Geometry check sheet. Reference: the model listing, model coordinates, mm. Coordinates: 2 decimals unless noted, no trailing zeros. Write each loop counter-clockwise with the first axis right and the second up, starting at its lowest first coordinate (ties: lowest second). Pieces come first, ordered by that corner, then holes. Notation, with made-up numbers: (20, 40.25) -> (62, 40.25) arc R9 cw to (62, 57.25) -> close; hole circle Ø10 at (36, 29). An arc over 180 degrees is marked (long way). Use a Markdown table: item, result.
Autodesk Inventor part; units mm, degrees
ref_plane "YZ Plane" through (0, 0, 0) normal (1, 0, 0) x (0, 1, 0)
ref_plane "XZ Plane" through (0, 0, 0) normal (0, 1, 0) x (-1, 0, 0)
ref_plane "XY Plane" through (0, 0, 0) normal (0, 0, 1) x (1, 0, 0)
sketch "Sketch1" plane through (0, 0, 0) normal (0, 0, 1) x (1, 0, 0)
  line L0 (0, 37.2) -> (5, 42.2)
  line L1 (37.2, 42.2) -> (42.2, 37.2)
  line L2 (42.2, 5) -> (37.2, 0)
  line L3 (5, 0) -> (0, 5)
  line L4 (0, 37.2) -> (0, 5)
  line L5 (37.2, 42.2) -> (5, 42.2)
  line L6 (42.2, 5) -> (42.2, 37.2)
  line L7 (5, 0) -> (37.2, 0)
  line L8 (0, 5) -> (0, 0)
  circle A0 centre (21.1, 21.1) radius 2.5
  circle A1 centre (5.6, 36.6) radius 1.5
  circle A2 centre (36.6, 36.6) radius 1.5
  circle A3 centre (36.6, 5.6) radius 1.5
  circle A4 centre (5.6, 5.6) radius 1.5
  dimension "d8" = 5
  dimension "d9" = 5
  dimension "d10" = 5
  dimension "d11" = 21.1
  dimension "d12" = 21.1
  dimension "d13" = 3
  dimension "d14" = 3
  dimension "d15" = 3
  dimension "d16" = 3
  dimension "d17" = 31
  dimension "d18" = 31
  dimension "d19" = 31
  dimension "d20" = 31
  dimension "d21" = 5.6
  dimension "d22" = 5.6
  dimension "d43" = 5.6
  dimension "d44" = 5.6
  dimension "d45" = 5.6
  dimension "d46" = 5.6
  dimension "d47" = 42.2
extrude "Extrusion1" add sketch "Sketch1" along normal blind 9.8
sketch "Sketch2" plane through (0, 0, 9.8) normal (0, 0, 1) x (1, 0, 0)
  circle A0 centre (21.1, 21.1) radius 2.5
  circle A1 centre (5.6, 5.6) radius 1.5
  circle A2 centre (36.6, 5.6) radius 1.5
  circle A3 centre (36.6, 36.6) radius 1.5
  circle A4 centre (5.6, 36.6) radius 1.5
  line L0 (5, 42.2) -> (0, 37.2)
  line L1 (0, 37.2) -> (0, 5)
  line L2 (0, 5) -> (5, 0)
  line L3 (5, 0) -> (37.2, 0)
  line L4 (37.2, 0) -> (42.2, 5)
  line L5 (42.2, 5) -> (42.2, 37.2)
  line L6 (42.2, 37.2) -> (37.2, 42.2)
  line L7 (37.2, 42.2) -> (5, 42.2)
  point P0 (0, 0)
fillet "Fillet1" radius 0.25 8 edges at (21.1, 42.2, 9.8) (39.7, 39.7, 9.8) (42.2, 21.1, 9.8) (39.7, 2.5, 9.8) (21.1, 0, 9.8) (2.5, 2.5, 9.8) (0, 21.1, 9.8) (2.5, 39.7, 9.8)
extrude "Extrusion2" add sketch "Sketch2" along normal blind 31
sketch "Sketch3" plane through (0, 0, 40.8) normal (0, 0, 1) x (1, 0, 0)
  circle A0 centre (21.1, 21.1) radius 2.5
  circle A1 centre (5.6, 36.6) radius 1.5
  circle A2 centre (36.6, 36.6) radius 1.5
  circle A3 centre (36.6, 5.6) radius 1.5
  circle A4 centre (5.6, 5.6) radius 1.5
  line L0 (5, 42.2) -> (0, 37.2)
  line L1 (0, 37.2) -> (0, 5)
  line L2 (0, 5) -> (5, 0)
  line L3 (5, 0) -> (37.2, 0)
  line L4 (37.2, 0) -> (42.2, 5)
  line L5 (42.2, 5) -> (42.2, 37.2)
  line L6 (42.2, 37.2) -> (37.2, 42.2)
  line L7 (37.2, 42.2) -> (5, 42.2)
  point P0 (0, 0)
fillet "Fillet2" radius 0.25 8 edges at (21.1, 42.2, 40.8) (39.7, 39.7, 40.8) (42.2, 21.1, 40.8) (39.7, 2.5, 40.8) (21.1, 0, 40.8) (2.5, 2.5, 40.8) (0, 21.1, 40.8) (2.5, 39.7, 40.8)
extrude "Extrusion3" add sketch "Sketch3" along normal blind 7.75
sketch "Sketch4" plane through (0, 0, 48.55) normal (0, 0, 1) x (1, 0, 0)
  circle A0 centre (21.1, 21.1) radius 2.5
  circle A1 centre (21.1, 21.1) radius 16
  point P0 (0, 0)
  dimension "d31" = 32
extrude "Extrusion4" cut sketch "Sketch4" against normal blind 0.6
sketch "Sketch5" plane through (21.1, 21.1, 47.95) normal (0, 0, 1) x (1, 0, 0)
  circle A0 centre (0, 0) radius 2.5
  circle A1 centre (0, 0) radius 16
  circle A2 centre (0, 0) radius 11
  point P0 (-21.1, -21.1)
  dimension "d35" = 22
extrude "Extrusion5" add sketch "Sketch5" along normal blind 2.2 contours A2
fillet "Fillet3" radius 0.5 1 edges at (10.1, 21.1, 50.15)
sketch "Sketch6" plane through (21.1, 21.1, 50.15) normal (0, 0, 1) x (1, 0, 0)
  circle A0 centre (0, 0) radius 2.5
  point P0 (-21.1, -21.1)
extrude "Extrusion6" add sketch "Sketch6" along normal blind 22.5
fillet "Fillet4" radius 0.5 1 edges at (18.6, 21.1, 72.65)
sketch "Sketch7" plane through (21.1, 21.1, 72.65) normal (0, 0, 1) x (1, 0, 0)
  circle A0 centre (0, 0) radius 2.6386
  point P0 (-21.1, -21.1)
extrude "Extrusion7" add sketch "Sketch7" along normal blind 15
sketch "Sketch8" plane through (21.1, 21.1, 87.65) normal (0, 0, 1) x (1, 0, 0)
  circle A0 centre (0, 0) radius 2
  circle A1 centre (0, 0) radius 4.7625
  point P0 (-21.1, -21.1)
  dimension "d50" = 9.525
extrude "Extrusion8" add sketch "Sketch8" along normal blind 12.7 contours A0 | A1
sketch "Sketch9" plane through (21.1, 21.1, 87.65) normal (0, 0, -1) x (-1, 0, 0)
  circle A0 centre (0, 0) radius 4.7625
  circle A1 centre (0, 0) radius 2.6386
  point P0 (21.1, -21.1)
extrude "Extrusion9" add sketch "Sketch9" along normal blind 12.7
sketch "Sketch10" plane through (0, 0, 0) normal (0, 0, -1) x (-1, 0, 0)
  circle A0 centre (-21.1, 21.1) radius 2.5
  circle A1 centre (-5.6, 5.6) radius 1.5
  circle A2 centre (-36.6, 5.6) radius 1.5
  circle A3 centre (-36.6, 36.6) radius 1.5
  circle A4 centre (-5.6, 36.6) radius 1.5
  line L0 (0, 37.2) -> (-5, 42.2)
  line L1 (-5, 42.2) -> (-37.2, 42.2)
  line L2 (-37.2, 42.2) -> (-42.2, 37.2)
  line L3 (-42.2, 37.2) -> (-42.2, 5)
  line L4 (-42.2, 5) -> (-37.2, 0)
  line L5 (-37.2, 0) -> (-5, 0)
  line L6 (-5, 0) -> (0, 5)
  line L7 (0, 5) -> (0, 37.2)
  circle A5 centre (-21.1, 21.1) radius 2
  circle A6 centre (-21.1, 21.1) radius 2.5
  circle A7 centre (-21.1, 21.1) radius 2.5
  point P0 (0, 0)
extrude "Extrusion10" cut sketch "Sketch10" against normal blind 72.8 contours A0 | A1 | A2 | A3 | A4 | L7 L6 L5 L4 L3 L2 L1 L0 | A5
sketch "Sketch12" plane through (21.1, 21.1, 72.8) normal (0, 0, -1) x (-1, 0, 0)
  circle A0 centre (0, 0) radius 2.6386
  point P0 (21.1, -21.1)
extrude "Extrusion11" cut sketch "Sketch12" against normal blind 16.7
sketch "Sketch13" plane through (21.1, 21.1, 100.35) normal (0, 0, 1) x (1, 0, 0)
  circle A0 centre (0, 0) radius 4.7625
  point P0 (-21.1, -21.1)
extrude "Extrusion12" cut sketch "Sketch13" against normal blind 5.08
properties part number "Nema 17 adapter"
Item 1: Section check A-A on x = 21.1. Record the boundary of the cut face in (y, z), then the cut area to 3 significant figures.
Answer block:
| item | result |
|---|---|
| outline | (16.34, 74.95) -> (18.46, 74.95) -> (18.46, 89.5) -> (23.74, 89.5) -> (23.74, 74.95) -> (25.86, 74.95) -> (25.86, 95.27) -> (16.34, 95.27) -> close |
| area | 117 mm^2 |
Item 2: Mould release check, pull along Y, two halves, no side actions. Record for faces 1 (the flat face through (21, 21, 89.5)), 2 (the flat face through (19, 19, 74.95)), 3 (the cylindrical face through (23.045, 22.883, 82.123)): +Y half, -Y half, draft (parallel to the pull), parting line (faces both ways), or undercut.
Answer block:
| item | result |
|---|---|
| face 1 | undercut |
| face 2 | draft |
| face 3 | undercut |
Item 3: Section check D-D on z = 91.75. Record the boundary of the cut face in (x, y) (1 decimal), then the cut area to 3 significant figures.
Answer block:
| item | result |
|---|---|
| outline | circle Ø9.5 at (21.1, 21.1) |
| area | 71.3 mm^2 |
Item 4: Thickness scan on L1, parallel to Y at x = 21, z = 89; L2, parallel to Y at x = 19.5, z = 78.25. Record the ranges inside material, lowest first. Write a range as [from, to].
Answer block:
| item | result |
|---|---|
| L1 | y = [16.34, 18.46], [23.74, 25.86] |
| L2 | y = [16.61, 19], [23.2, 25.59] |
Item 5: Section check C-C on z = 78.75. Record the boundary of the cut face in (x, y) (1 decimal), then the cut area to 3 significant figures.
Answer block:
| item | result |
|---|---|
| outline | circle Ø9.5 at (21.1, 21.1); hole circle Ø5.3 at (21.1, 21.1) |
| area | 49.4 mm^2 |
Item 6: Depth check by flat-ended pin: P1, Ø1.5, axis at x = 17.5, z = 92, coming from the -Y side; P2, Ø3, axis at x = 22.5, z = 83.5, coming from the -Y side; P3, Ø1.6, axis at x = 20, y = 20, coming from the -Z side; P4, Ø1.5, axis at x = 19.5, z = 80.5, coming from the -Y side. Enter the tip coordinate at first touch or a pass-through.
Answer block:
| item | result |
|---|---|
| P1 | stops at y = 17.28 |
| P2 | stops at y = 16.34 |
| P3 | stops at z = 89.5 |
| P4 | stops at y = 16.41 |
